The listing builds one solid part. Answer for the finished solid, in the listing's coordinates (mm). Face numbers are marked on the shaded views. A direction names the side the tool comes from. Round coordinates to 2 decimals unless told otherwise and drop trailing zeros. Write each loop counter-clockwise with the first axis right and the second up, starting at its lowest first coordinate (ties: lowest second). Pieces come first, ordered by that corner, then holes. Notation, with made-up numbers: (-40, -17) - (-1, -17) arc R31 cw to (-1, 14) - close; hole circle Ø5 at (9.25, -34). An arc over 180 degrees is marked (long way). Use a Markdown table: item, result. Add a question column.
1) Find the intervals of material crossed by probe 1 along X at (y, z) = (2.5, 6); probe 2 along Y at (x, z) = (21, 7); probe 3 along X at (y, z) = (40.5, 7.5), in increasing order. Write a range as from..to.
2) A cutting plane is placed at A-A (z = 9.7). Give the vertices of the cut face in (x, y), then the cut area to 3 significant figures.
3) A cutting plane is placed at D-D (z = 2.75). Give the vertices of the cut face in (x, y), then the cut area to 3 significant figures.
4) Determine the mould class of the marked faces 3, 4, 5 and 6 for opening direction X: +X half, -X half, draft (parallel to the pull), parting line (faces both ways), or undercut.
5) A tool of negligible diameter and unlimited length cuts with its end or side. For the marked faces 1 and 2, from which of +Z, -Z, +X, -X, +Y, -Y can it reach the whole face along a straight path? Write none if from no direction.
6) A cutting plane is placed at B-B (y = 25). Give the vertices of the cut face in (x, z), then the cut area to 3 significant figures.
7) Each of these flat-tipped pins is pushed along its axis until it touches: P1, Ø5, axis at y = 39, z = 7, coming from the -X side; P2, Ø2, axis at x = 13, z = 9.7, coming from the +Y side. Where does it stop, or does it pass through?
8) A cutting plane is placed at C-C (x = 27). Give the vertices of the cut face in (y, z).
```python
from build123d import *

# Parameters (mm, degrees)
SKETCH1_W           = 54
SKETCH1_H           = 59
SKETCH1_W_2         = 40
SKETCH1_H_2         = 52
BOSS_EXTRUDE1_DEPTH = 12
SKETCH2_R           = 1.85
CUT_EXTRUDE1_DEPTH  = 10
SKETCH3_R           = 1.85
CUT_EXTRUDE2_DEPTH  = 10


with BuildPart() as part:
    # Sketch1 → Boss-Extrude1 (new body)
    with BuildSketch(Plane.XY):
        with Locations((27, 29.5)):
            Rectangle(SKETCH1_W, SKETCH1_H)
        with Locations((27, 29.5)):
            Rectangle(SKETCH1_W_2, SKETCH1_H_2, mode=Mode.SUBTRACT)
    extrude(amount=BOSS_EXTRUDE1_DEPTH)

    # Sketch2 → Cut-Extrude1 (cut)
    with BuildSketch(Plane(origin=(0, 59, 0), x_dir=(1, 0, 0), z_dir=(0, 1, 0))):
        with Locations(Location((13, -9.7, 0), (0, 0, 180))):
            Circle(SKETCH2_R)
        with Locations(Location((41, -9.7, 0), (0, 0, 180))):
            Circle(SKETCH2_R)
        with Locations(Location((27, -9.7, 0), (0, 0, 180))):
            Circle(SKETCH2_R)
    extrude(amount=-CUT_EXTRUDE1_DEPTH, mode=Mode.SUBTRACT)

    # Sketch3 → Cut-Extrude2 (cut)
    with BuildSketch(Plane.XZ):
        with Locations(Location((12.75, 6, 0), (0, 0, 270))):
            Circle(SKETCH3_R)
        with Locations(Location((41.25, 6, 0), (0, 0, 90))):
            Circle(SKETCH3_R)
    extrude(amount=-CUT_EXTRUDE2_DEPTH, mode=Mode.SUBTRACT)


solid = part.part
```
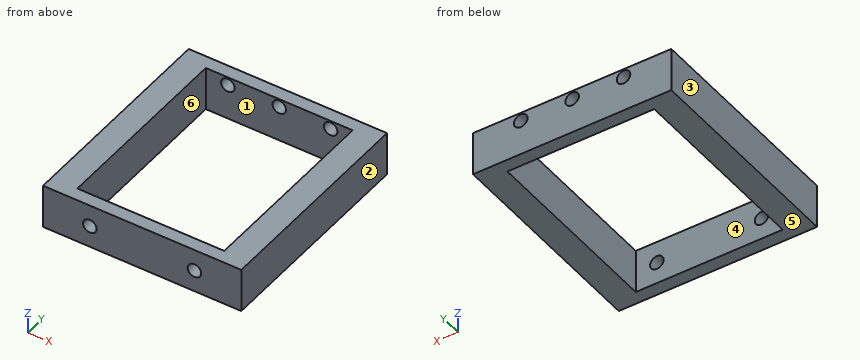
Entries:
| question | item | result |
|---|---|---|
| 1 | probe 1 | x = 0..10.9, 14.6..39.4, 43.1..54 |
| 1 | probe 2 | y = 0..3.5, 55.5..59 |
| 1 | probe 3 | x = 0..7, 47..54 |
| 2 | outline | (0, 0) - (54, 0) - (54, 59) - (42.85, 59) - (42.85, 55.5) - (47, 55.5) - (47, 3.5) - (7, 3.5) - (7, 55.5) - (11.15, 55.5) - (11.15, 59) - (0, 59) - close; (14.85, 55.5) - (25.15, 55.5) - (25.15, 59) - (14.85, 59) - close; (28.85, 55.5) - (39.15, 55.5) - (39.15, 59) - (28.85, 59) - close |
| 2 | area | 1,070 mm² |
| 3 | outline | (0, 0) - (54, 0) - (54, 59) - (0, 59) - close; hole (7, 3.5) - (47, 3.5) - (47, 55.5) - (7, 55.5) - close |
| 3 | area | 1,110 mm² |
| 4 | face 3 | -X half |
| 4 | face 4 | undercut |
| 4 | face 5 | draft |
| 4 | face 6 | undercut |
| 5 | face 1 | +Z, -Z |
| 5 | face 2 | +Z, -Z, +X, +Y, -Y |
| 6 | outline | (0, 0) - (7, 0) - (7, 12) - (0, 12) - close; (47, 0) - (54, 0) - (54, 12) - (47, 12) - close |
| 6 | area | 168 mm² |
| 7 | P1 | stops at x = 0 |
| 7 | P2 | stops at y = 3.5 |
| 8 | outline | (0, 0) - (3.5, 0) - (3.5, 12) - (0, 12) - close; (55.5, 0) - (59, 0) - (59, 7.85) - (55.5, 7.85) - close; (55.5, 11.55) - (59, 11.55) - (59, 12) - (55.5, 12) - close |
